Check sheet for the modelled part. Datum: model origin and axes. Units: mm. A direction names the side the tool comes from. Give positions to 0.01 mm unless a question says otherwise; leave off trailing zeros. Loops run counter-clockwise (first coordinate to the right, second up) from the corner with the lowest first, then second, coordinate; pieces in that order, holes last. Notation, with made-up numbers: M 88,89 L 131,89 A30 cw 131,128 Z; hole C 63,49.5 d2. An arc over 180 degrees is marked long. One line per question, with ' | ' between items. Start each with the question number.
from build123d import *

# Parameters (mm, degrees)
F0_W     = 76.2
F0_H     = 19.05
F0_W_2   = 19.05
F0_H_2   = 38.1
F0_R     = 17.4625
F0_R_2   = 6.35
F1_DEPTH = 19.05
F2_DEPTH = 9.525


with BuildPart() as f1:
    # F0 (on Front) → F1 (new body)
    with BuildSketch(Plane.XZ):
        Polygon((-489.430563, 76.2), (-540.230563, 76.2), (-540.230563, 95.25), (-591.030563, 95.25), (-599.913724, 95.25), (-613.971884, 125.397822), (-596.706721, 133.4487), (-618.175729, 179.489136), (-635.440892, 171.438258), (-656.9099, 217.478693), (-639.644736, 225.529571), (-661.113744, 271.570007), (-678.378907, 263.519129), (-699.847915, 309.559564), (-682.582752, 317.610442), (-704.051759, 363.650878), (-721.316923, 355.6), (-743.430563, 355.6), (-997.430563, 127), (-997.430563, 0), (-591.030563, 0), (342.419437, 0), (371.914191, 0), (392.43009, 43.996488), (447.87154, 162.891061), (502.200551, 162.891061), (676.47154, 162.891061), (676.47154, 239.091061), (676.47154, 258.141061), (625.67154, 258.141061), (625.67154, 239.091061), (573.840427, 239.091061), (573.840427, 258.141061), (523.040427, 258.141061), (523.040427, 239.091061), (472.240427, 239.091061), (472.240427, 258.141061), (421.440427, 258.141061), (421.440427, 239.091061), (399.326786, 239.091061), (382.061623, 247.141939), (360.592615, 201.101503), (377.857779, 193.050626), (356.388771, 147.01019), (339.123608, 155.061068), (317.6546, 109.020632), (334.919763, 100.969754), (324.841751, 79.357387), (323.369437, 76.2), (272.569437, 76.2), (272.569437, 95.25), (221.769437, 95.25), (221.769437, 76.2), (170.969437, 76.2), (170.969437, 95.25), (120.169437, 95.25), (120.169437, 76.2), (69.369437, 76.2), (69.369437, 95.25), (18.569437, 95.25), (18.569437, 76.2), (-32.230563, 76.2), (-32.230563, 95.25), (-83.030563, 95.25), (-83.030563, 76.2), (-133.830563, 76.2), (-133.830563, 95.25), (-184.630563, 95.25), (-184.630563, 76.2), (-235.430563, 76.2), (-235.430563, 95.25), (-286.230563, 95.25), (-286.230563, 76.2), (-337.030563, 76.2), (-337.030563, 95.25), (-387.830563, 95.25), (-387.830563, 76.2), (-438.630563, 76.2), (-438.630563, 95.25), (-489.430563, 95.25), align=None)
        with Locations((-705.330563, 34.925)):
            Rectangle(F0_W, F0_H, mode=Mode.SUBTRACT)
        with Locations((-581.505563, 44.45)):
            Rectangle(F0_W_2, F0_H_2, mode=Mode.SUBTRACT)
        with Locations((-932.089063, 57.15)):
            Circle(F0_R, mode=Mode.SUBTRACT)
        with Locations((-705.330563, 82.55)):
            Circle(F0_R_2, mode=Mode.SUBTRACT)
        with Locations((-159.243268, 44.45)):
            Rectangle(F0_W_2, F0_H_2, mode=Mode.SUBTRACT)
        with Locations((351.944437, 44.45)):
            Rectangle(F0_W_2, F0_H_2, mode=Mode.SUBTRACT)
        Polygon((-832.288567, 215.839342), (-845.030563, 230.0007), (-788.385133, 280.968682), (-775.643137, 266.807325), align=None, mode=Mode.SUBTRACT)
        with Locations((411.915427, 200.991061)):
            Rectangle(F0_W_2, F0_H_2, mode=Mode.SUBTRACT)
        with Locations((549.47154, 191.466061)):
            Rectangle(F0_W, F0_H, mode=Mode.SUBTRACT)
        with Locations((641.54654, 200.991061)):
            Rectangle(F0_W_2, F0_H_2, mode=Mode.SUBTRACT)
    extrude(amount=F1_DEPTH)

    # F0 (on Front) → F2 (join)
    with BuildSketch(Plane.XZ):
        with Locations((-932.089063, 57.15)):
            Circle(F0_R)
        with Locations((-932.089063, 57.15)):
            Circle(F0_R_2, mode=Mode.SUBTRACT)
    extrude(amount=F2_DEPTH)


solid = f1.part
Q1. Depth check by flat-ended pin: P1, Ø9.5, axis at x = -475, y = -13.5, coming from the +Z side; P2, Ø5.5, axis at y = -5.5, z = 31, coming from the +X side; P3, Ø1, axis at x = -807.5, y = -5, coming from the +Z side. Enter the tip coordinate at first touch or a pass-through.
Q2. Cross-section at B-B (x = 299). Record the cut outline in (y, z), and give its area (3 significant figures).
Q3. Access from +Z, -Z, +X, -X, +Y, -Y to the whole of each face (thin tool, end or side, straight path). Record for faces 4 (the flat face through (-803.57, -9.39, 241.68)), 5 (the flat face through (-358, 0, 63)), 6 (the flat face through (-925, -9.525, 57)).
Q4. Material ranges on probe 1 along Z at (x, y) = (-151, -5); probe 2 along X at (y, z) = (-2.5, 267) (1 decimal); probe 3 along X at (y, z) = (-10.5, 222) (3 decimals), recorded low to high. Write a range as from..to.
Q5. Draft check along X on faces 1 (the cylindrical face through (-949.535, -14.221, 57.918)), 2 (the flat face through (-350, -19.05, 61)), 3 (the flat face through (-868.65, -9.39, 242.9)). Enter one of: released by +X, released by -X, zero draft, split by the parting line, or undercut.
Q6. Cross-section at A-A (y = -16). State how many separate pieces and enclosed holes the cut face has, and give its area (3 significant figures).
Solved:
1) P1: stops at z = 95.25 | P2: stops at x = 387.65 | P3: stops at z = 298.39
2) outline: M -19.05,0 L 0,0 L 0,76.2 L -19.05,76.2 Z | area: 1,450 mm²
3) face 4: +Y, -Y | face 5: +Z, -Z, +X, -X, +Y | face 6: -Y
4) probe 1: z = 0..25.4, 63.5..95.25 | probe 2: x = -841.9..-803.9, -775.8..-680, -670.9..-659 | probe 3: x = -891.875..-837.832, -825.442..-647.214, 370.338..676.472
5) face 1: undercut | face 2: zero draft | face 3: released by -X
6) separate pieces: 1 | enclosed holes: 10 | area: 209,000 mm²
